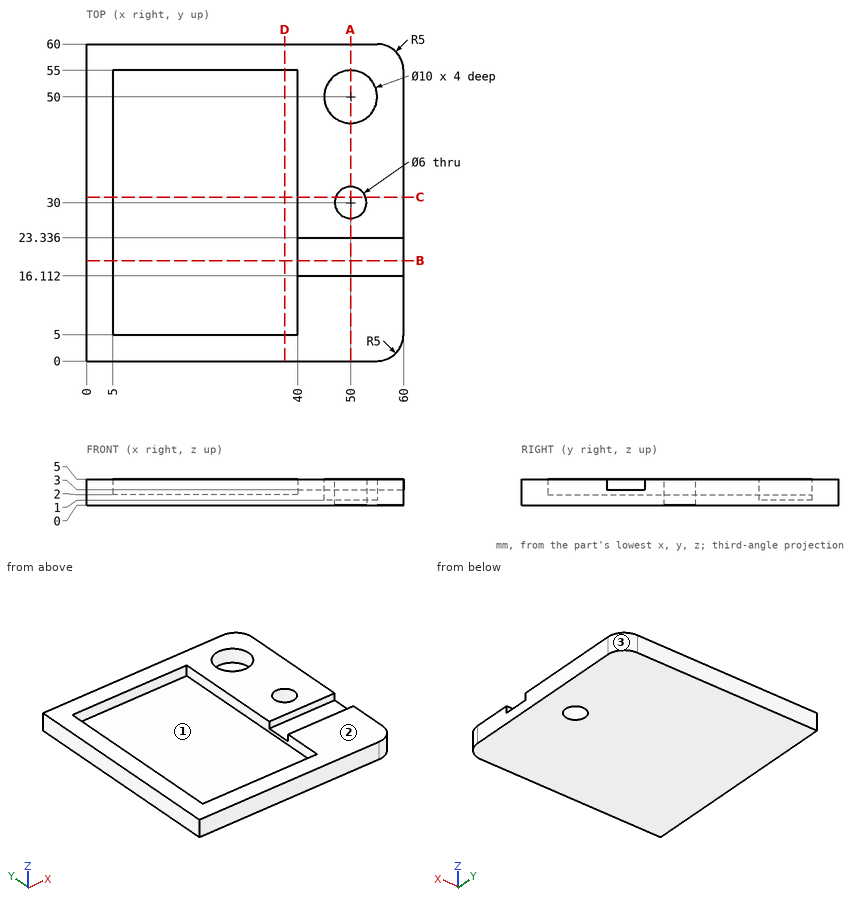
Verification items for this drawing (mm, ordinates from the low corner). Coordinates: 2 decimals unless noted, no trailing zeros. Order: outer loops, then holes, each group sorted by start corner. A loop starts at its lowest first (then second) coordinate and runs counter-clockwise, first axis right, second up. Notation, with made-up numbers: (-12.5, 5) - (28.5, 5) arc R24 ccw to (28.5, 25) - close; hole circle Ø7 at (-17, 19). An arc over 180 degrees is marked (long way). Answer as a JSON object with one key per item and string values. Group by question number.
Item 1: Sectioned sample at D-D, the plane x = 37.5. Record the cut outline in (y, z).
Item 2: Sectioned sample at C-C, the plane y = 31. Record the cut outline in (x, z).
Item 3: Draft check along X on the marked faces 1, 2 and 3. Enter one of: +X half, -X half, draft (parallel to the pull), parting line (faces both ways), or undercut.
Item 4: Depth check by flat-ended pin: pin 1 Ø5 at (x, y) = (50.5, 49.5) entering from +Z; pin 2 Ø2 at (x, y) = (54.5, 18.5) entering from +Z; pin 3 Ø3 at (x, y) = (27, 25.5) entering from +Z. Enter the tip coordinate at first touch or a pass-through.
Item 5: Sectioned sample at B-B, the plane y = 19. Record the cut outline in (x, z), and give its area (3 significant figures).
Item 6: Scan lines: probe 1 along Y at (x, z) = (50, 3.4) (1 decimal); probe 2 along Y at (x, z) = (18, 4.5); probe 3 along Y at (x, z) = (42, 4.65) (1 decimal). Record each from-to range of solid material in increasing order.
Item 7: Sectioned sample at A-A, the plane x = 50. Record the cut outline in (y, z) (1 decimal).
Resolved:
{
 "1": {"outline": "(0, 0) - (60, 0) - (60, 5) - (55, 5) - (55, 2) - (5, 2) - (5, 5) - (0, 5) - close"},
 "2": {"outline": "(0, 0) - (47.17, 0) - (47.17, 5) - (40, 5) - (40, 2) - (5, 2) - (5, 5) - (0, 5) - close; (52.83, 0) - (60, 0) - (60, 5) - (52.83, 5) - close"},
 "3": {"face 1": "undercut", "face 2": "draft", "face 3": "+X half"},
 "4": {"pin 1": "z = 1", "pin 2": "z = 3", "pin 3": "z = 2"},
 "5": {"outline": "(0, 0) - (60, 0) - (60, 3) - (40, 3) - (40, 2) - (5, 2) - (5, 5) - (0, 5) - close", "area": "155 mm^2"},
 "6": {"probe 1": "0 to 16.1, 23.3 to 27, 33 to 45, 55 to 60", "probe 2": "0 to 5, 55 to 60", "probe 3": "0 to 16.1, 23.3 to 60"},
 "7": {"outline": "(0, 0) - (27, 0) - (27, 5) - (23.3, 5) - (23.3, 3) - (16.1, 3) - (16.1, 5) - (0, 5) - close; (33, 0) - (60, 0) - (60, 5) - (55, 5) - (55, 1) - (45, 1) - (45, 5) - (33, 5) - close"}
}
